Print and shaded views of the part. All mm, measured from the part's lowest x, y and z. Give positions to 0.01 mm unless a question says otherwise; leave off trailing zeros. Write each loop counter-clockwise with the first axis right and the second up, starting at its lowest first coordinate (ties: lowest second). Pieces come first, ordered by that corner, then holes.
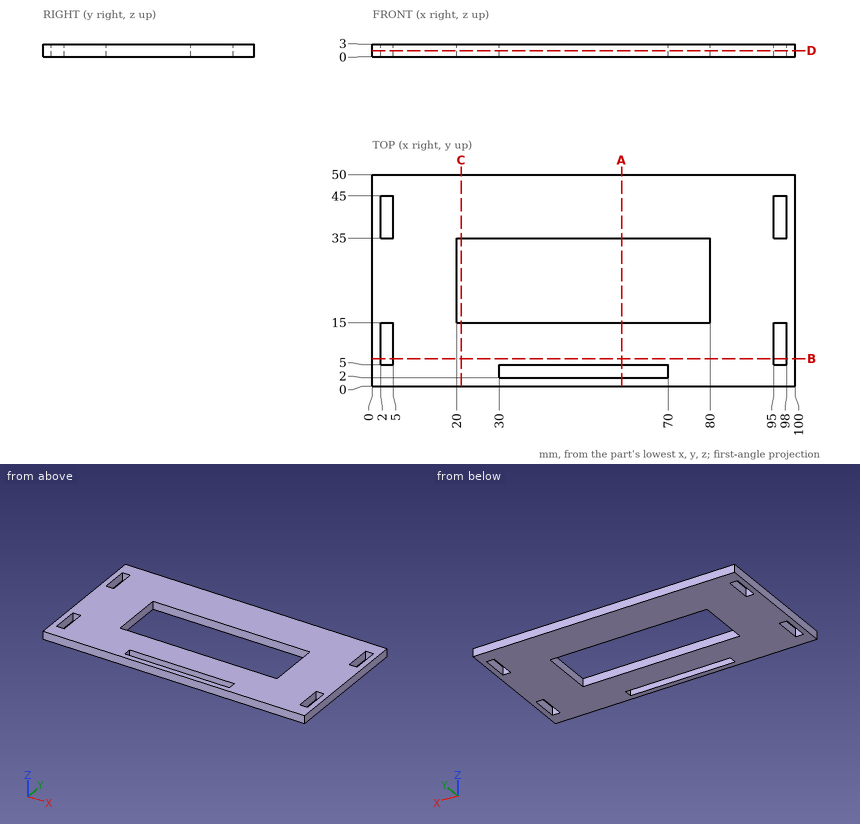
1. Saw through at B-B on y = 6.5. Give the cut face in (x, z), plus the area to 3 significant figures.
2. Drill centre lines: line 1 along Y through (x, z) = (39, 0.7); line 2 along X through (y, z) = (40, 1.9); line 3 along Y through (x, z) = (23, 2.5). Where is each one in solid material? Low to high.
3. Saw through at A-A on x = 59. Give the cut face in (y, z).
4. Drop a flat-ended pin along its axis: pin 1 (5 mm diameter, centred on x = 77, y = 28, fed in from +Z). Give the stop position or say it passes through.
5. Saw through at C-C on x = 21. Give the cut face in (y, z), plus the area to 3 significant figures.
6. Saw through at D-D on z = 1.45. Give the cut face in (x, y).
Outcome:
1. outline: (0, 0) - (2, 0) - (2, 3) - (0, 3) - close; (5, 0) - (95, 0) - (95, 3) - (5, 3) - close; (98, 0) - (100, 0) - (100, 3) - (98, 3) - close
1. area: 282 mm2
2. line 1: y = 0 to 2, 5 to 15, 35 to 50
2. line 2: x = 0 to 2, 5 to 95, 98 to 100
2. line 3: y = 0 to 15, 35 to 50
3. outline: (0, 0) - (2, 0) - (2, 3) - (0, 3) - close; (5, 0) - (15, 0) - (15, 3) - (5, 3) - close; (35, 0) - (50, 0) - (50, 3) - (35, 3) - close
4. pin 1: passes through
5. outline: (0, 0) - (15, 0) - (15, 3) - (0, 3) - close; (35, 0) - (50, 0) - (50, 3) - (35, 3) - close
5. area: 90.0 mm2
6. outline: (0, 0) - (100, 0) - (100, 50) - (0, 50) - close; hole (2, 5) - (5, 5) - (5, 15) - (2, 15) - close; hole (2, 35) - (5, 35) - (5, 45) - (2, 45) - close; hole (20, 15) - (80, 15) - (80, 35) - (20, 35) - close; hole (30, 2) - (70, 2) - (70, 5) - (30, 5) - close; hole (95, 5) - (98, 5) - (98, 15) - (95, 15) - close; hole (95, 35) - (98, 35) - (98, 45) - (95, 45) - close
